from build123d import *

# Parameters (mm, degrees)
BOSS_EXTRUDE1_DEPTH = 50
SKETCH2_R           = 13.5
CUT_EXTRUDE1_DEPTH  = 32
SKETCH3_R           = 4.15
CUT_EXTRUDE2_DEPTH  = 59.454827457
CUT_EXTRUDE3_DEPTH  = 59.454827457


with BuildPart() as part:
    # Sketch1 → Boss-Extrude1 (new body)
    with BuildSketch(Plane(origin=(0, 0, 0), x_dir=(1, 0, 0), z_dir=(0, 1, 0))):
        with BuildLine():
            ThreePointArc((0, 20), (20, 0), (0, -20))
            ThreePointArc((0, -20), (-22.604078238, 0), (0, 20))
        make_face()
    extrude(amount=BOSS_EXTRUDE1_DEPTH)

    # Sketch2 → Cut-Extrude1 (cut)
    with BuildSketch(Plane.XZ):
        with Locations(Location((0, 0, 0), (0, 0, 270))):
            Circle(SKETCH2_R)
    extrude(amount=-CUT_EXTRUDE1_DEPTH, mode=Mode.SUBTRACT)

    # Sketch3 → Cut-Extrude2 (cut, through all)
    with BuildSketch(Plane(origin=(0, 50, 0), x_dir=(1, 0, 0), z_dir=(0, 1, 0))):
        with Locations(Location((0, 0, 0), (0, 0, 270))):
            Circle(SKETCH3_R)
    extrude(amount=-CUT_EXTRUDE2_DEPTH, mode=Mode.SUBTRACT)

    # Sketch4 → Cut-Extrude3 (cut, through all)
    with BuildSketch(Plane(origin=(0, 50, 0), x_dir=(1, 0, 0), z_dir=(0, 1, 0))):
        with BuildLine():
            Line((-18.4, 7.5), (-18.4, 2.107130751))
            ThreePointArc((-18.4, 2.107130751), (-19, 0), (-18.4, -2.107130751))
            Line((-18.4, -2.107130751), (-18.4, -7.5))
            Line((-18.4, -7.5), (-5.6, -7.5))
            Line((-5.6, -7.5), (-5.6, 7.5))
            Line((-5.6, 7.5), (-18.4, 7.5))
        make_face()
    extrude(amount=-CUT_EXTRUDE3_DEPTH, mode=Mode.SUBTRACT)


solid = part.part
Check sheet for the modelled part. Datum: model origin and axes. Units: mm. A direction names the side the tool comes from. Coordinates: 2 decimals unless noted, no trailing zeros. Loops run counter-clockwise (first coordinate to the right, second up) from the corner with the lowest first, then second, coordinate; pieces in that order, holes last. Notation, with made-up numbers: (-28, -32.75) -> (18, -32.75) arc R12 cw to (18, -17.75) -> close; hole circle Ø4 at (-10, -34.5). An arc over 180 degrees is marked (long way). Write item = value, one per line. Start each with the question number.
1. Material ranges on line 1 (X direction, y = 46, z = 0); line 2 (X direction, y = 23, z = 0); line 3 (Z direction, x = 9, y = 18), recorded low to high.
2. Depth check by flat-ended pin: P1, Ø4.5, axis at y = 18, z = -5, coming from the +X side; P2, Ø12, axis at x = 8.5, y = 33, coming from the +Z side; P3, Ø2, axis at y = 32.5, z = 5, coming from the -X side; P4, Ø5, axis at x = 0, z = 0, coming from the -Y side. Enter the tip coordinate at first touch or a pass-through.
3. Draft check along X on faces 1 (the cylindrical face through (20, 25, 0)), 2 (the flat face through (-10.5, 0, -9.2)), 3 (the cylindrical face through (13.49, 15.78, -0.48)). Enter one of: released by +X, released by -X, zero draft, split by the parting line, or undercut.
4. Section check A-A on z = 0. Record the cut outline in (x, y).
5. Section check D-D on y = 38. Record the cut outline in (x, z).
6. Section check C-C on x = -3. Record the cut outline in (y, z), then the cut area to 3 significant figures.
7. Tool access check on faces 4 (the flat face through (4, 32, -3)), 5 (the flat face through (-13, 31, -7.5)), 6 (the flat face through (-1, 50, 4.2)). Record the directions out of +Z, -Z, +X, -X, +Y, -Y that give a thin tool (end or side, any length) a straight path to the whole face; none if there is none.
8. Section check B-B on y = 9.5. Record the cut outline in (x, z).
Responses:
q1.line_1 = -22.6 to -19, -5.6 to -4.15, 4.15 to 20
q1.line_2 = -22.6 to -19, 13.5 to 20
q1.line_3 = -17.86 to -10.06, 10.06 to 17.86
q2.P1 = 19.81
q2.P2 = 19.84
q2.P3 = -22.2
q2.P4 = through
q3.face_1 = released by +X
q3.face_2 = zero draft
q3.face_3 = undercut
q4.outline = (-22.6, 0) -> (-19, 0) -> (-19, 50) -> (-22.6, 50) -> close; (-5.6, 32) -> (-4.15, 32) -> (-4.15, 50) -> (-5.6, 50) -> close; (4.15, 32) -> (13.5, 32) -> (13.5, 0) -> (20, 0) -> (20, 50) -> (4.15, 50) -> close
q5.outline = (0, -20) arc R20 ccw to (0, 20) arc R20.15 ccw (long way) to start; hole (-18.4, -7.5) -> (-5.6, -7.5) -> (-5.6, 7.5) -> (-18.4, 7.5) -> (-18.4, 2.11) arc R4 ccw to (-18.4, -2.11) -> close; hole circle Ø8.3 at (0, 0)
q6.outline = (0, -20.14) -> (50, -20.14) -> (50, -2.87) -> (32, -2.87) -> (32, -13.16) -> (0, -13.16) -> close; (0, 13.16) -> (32, 13.16) -> (32, 2.87) -> (50, 2.87) -> (50, 20.14) -> (0, 20.14) -> close
q6.area = 1,070 mm2
q7.face_4 = -Y
q7.face_5 = +Y, -Y
q7.face_6 = +Z, -Z, +X, -X, +Y
q8.outline = (0, -20) arc R20 ccw to (0, 20) arc R20.15 ccw (long way) to start; hole (-18.4, -7.5) -> (-11.22, -7.5) arc R13.5 ccw (long way) to (-11.22, 7.5) -> (-18.4, 7.5) -> (-18.4, 2.11) arc R4 ccw to (-18.4, -2.11) -> close
